```python
from build123d import *

# Parameters (mm, degrees)
SKETCH3_R           = 3.6
BOSS_EXTRUDE1_DEPTH = 6.5
SKETCH4_R           = 2.5
BOSS_EXTRUDE2_DEPTH = 2.5
BOSS_EXTRUDE3_START = 2.5
SKETCH5_R           = 2.5
BOSS_EXTRUDE3_DEPTH = 2.5
CHAMFER1_SIZE       = 0.5


with BuildPart() as part:
    # Sketch3 → Boss-Extrude1 (new body)
    with BuildSketch(Plane.XY):
        with Locations(Location((0, 0, 0), (0, 0, 180))):
            Circle(SKETCH3_R)
    extrude(amount=BOSS_EXTRUDE1_DEPTH)

    # Sketch4 → Boss-Extrude2 (add)
    with BuildSketch(Plane.XY):
        Circle(SKETCH4_R)
    extrude(amount=-BOSS_EXTRUDE2_DEPTH)

    # Sketch5 → Boss-Extrude3 (add)
    with BuildSketch(Plane.XY.offset(6.5).offset(BOSS_EXTRUDE3_START)):
        Circle(SKETCH5_R)
    extrude(amount=-BOSS_EXTRUDE3_DEPTH)

    # Chamfer1
    chamfer1_edges = [part.edges().sort_by_distance(p)[0] for p in [
        (-2.5, 0, -2.5),
    ]]
    chamfer(chamfer1_edges, length=CHAMFER1_SIZE)


solid = part.part
```
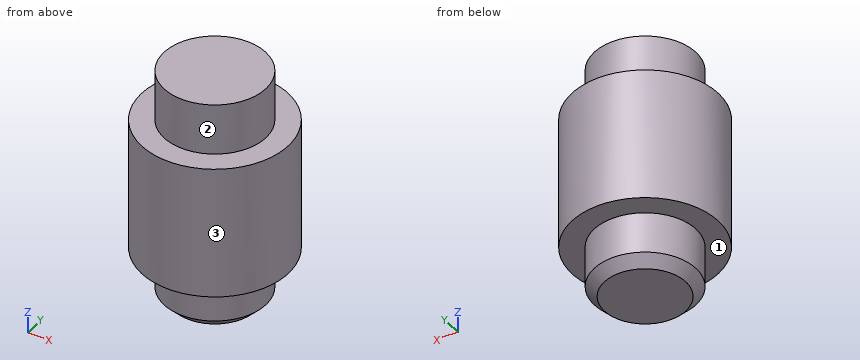
Input: part model. Units: mm. Frame: model coordinates. Face numbers are marked on the shaded views. A direction names the side the tool comes from. Round coordinates to 2 decimals unless told otherwise and drop trailing zeros. Write each loop counter-clockwise with the first axis right and the second up, starting at its lowest first coordinate (ties: lowest second). Pieces come first, ordered by that corner, then holes. Notation, with made-up numbers: (61.5, -4.75) - (77.5, -4.75) arc R13 cw to (77.5, 15.25) - close; hole circle Ø7 at (50, -4). An arc over 180 degrees is marked (long way). Write item = value, one per line.
(1) Contact query for a flat-ended pin moving along its axis: pin 1 Ø1 at (x, z) = (1.5, 0.5) entering from +Y. Output: stop coordinate, or through.
Geometry check:
pin_1 = 3.46
(2) Section query C-C on z = 2. Output: boundary loops of the cut face in (x, y).
Geometry check:
outline = circle Ø7.2 at (0, 0)
(3) Section query A-A on x = 0. Output: boundary loops of the cut face in (y, z), then the cut area to 4 significant figures.
Geometry check:
outline = (-3.6, 0) - (-2.5, 0) - (-2.5, -2) - (-2, -2.5) - (2, -2.5) - (2.5, -2) - (2.5, 0) - (3.6, 0) - (3.6, 6.5) - (2.5, 6.5) - (2.5, 9) - (-2.5, 9) - (-2.5, 6.5) - (-3.6, 6.5) - close
area = 71.55 mm^2
(4) Material intervals for probe 1 along Z at (x, y) = (-3, -1.5); probe 2 along X at (y, z) = (-1.5, -1); probe 3 along Y at (x, z) = (-2.75, 6.25), sorted ascending.
Geometry check:
probe_1 = 0 to 6.5
probe_2 = -2 to 2
probe_3 = -2.32 to 2.32
(5) Access query for the marked faces 1, 2 and 3. Directions: +Z, -Z, +X, -X, +Y, -Y. A direction counts if a zero-diameter tool reaches every point of the face in a straight line with its end or side. Return the directions, or none.
Geometry check:
face_1 = -Z
face_2 = +Z
face_3 = +Z, -Z
(6) Section query D-D on z = 7.25. Output: boundary loops of the cut face in (x, y), then the cut area to 3 significant figures.
Geometry check:
outline = circle Ø5 at (0, 0)
area = 19.6 mm^2
